For this review, take the finished solid that the model builds, in its own axes (mm). A direction names the side the tool comes from. Give positions to 0.01 mm unless a question says otherwise; leave off trailing zeros.
1) Machinability: for faces 1 (the face through (0, 10, 0)), 2 (the face through (-2.373, 3.451, 3.095)), which of the approach directions +Z, -Z, +X, -X, +Y, -Y give a long, thin tool a straight path to every point of the face, cutting with its end or side? Answer none if there is none.
2) Wall thickness on line 1 along X through (y, z) = (4.25, 3.25); line 2 along Y through (x, z) = (-2.5, 1.5); line 3 along X through (y, z) = (6, -4.25): over which ranges is each line inside the solid? List them lowest first.
3) For P1, Ø1, axis at y = 3.5, z = -8, coming from the -X side; P2, Ø4, axis at x = -7, y = 6.5, coming from the -Z side; P3, Ø5, axis at y = 6.5, z = -3.5, coming from the -X side, all flat-tipped, find the tip position at first contact; note any pin that passes through.
from build123d import *

# Parameters (mm, degrees)
SKETCH1_R           = 15
BOSS_EXTRUDE1_DEPTH = 10
SKETCH2_R           = 3.9
CUT_EXTRUDE1_DEPTH  = 7
FILLET1_R           = 10


with BuildPart() as part:
    # Sketch1 → Boss-Extrude1 (new body)
    with BuildSketch(Plane(origin=(0, 0, 0), x_dir=(1, 0, 0), z_dir=(0, 1, 0))):
        with Locations(Location((0, 0, 0), (0, 0, 270))):
            Circle(SKETCH1_R)
    extrude(amount=BOSS_EXTRUDE1_DEPTH)

    # Sketch2 → Cut-Extrude1 (cut)
    with BuildSketch(Plane.XZ):
        with Locations(Location((0, 0, 0), (0, 0, 270))):
            Circle(SKETCH2_R)
    extrude(amount=-CUT_EXTRUDE1_DEPTH, mode=Mode.SUBTRACT)

    # Fillet1
    fillet1_edges = [part.edges().sort_by_distance(p)[0] for p in [
        (0, 0, -15),
    ]]
    fillet(fillet1_edges, radius=FILLET1_R - 0.0001)  # a hair under: the kernel refuses the full size


solid = part.part
Results list:
1. face 1: +Z, -Z, +X, -X, +Y
1. face 2: -Y
2. line 1: x = -12.77 to -2.16, 2.16 to 12.77
2. line 2: y = 7 to 10
2. line 3: x = -13.51 to 13.51
3. P1: stops at x = -10.38
3. P2: stops at z = -13.71
3. P3: stops at x = -14.75
